Can you work these out from the model? Positions are in its coordinate system, mm. Face numbers are marked on the shaded views. A direction names the side the tool comes from. Give positions to 0.01 mm unless a question says otherwise; leave off trailing zeros. Order: outer loops, then holes, each group sorted by start corner. A loop starts at its lowest first (then second) coordinate and runs counter-clockwise, first axis right, second up. Notation, with made-up numbers: (25.25, 87) - (70.25, 87) arc R5 ccw to (70.25, 94) - close; hole circle Ø2 at (10, 21.25). An arc over 180 degrees is marked (long way). Answer as a JSON object with one key per item and string values.
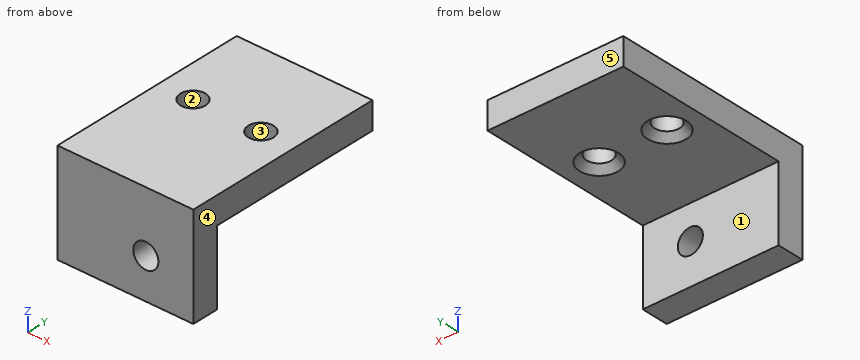
```python
from build123d import *

# Parameters (mm, degrees)
BOSS_EXTRUDE1_DEPTH = 10
SKETCH2_R           = 1.85
CUT_EXTRUDE1_DEPTH  = 30.949958264
BOSS_EXTRUDE2_DEPTH = 10
SKETCH4_R           = 1.85
CUT_EXTRUDE2_DEPTH  = 30.949958264
CHAMFER1_SIZE       = 1


with BuildPart() as part:
    # Sketch1 → Boss-Extrude1 (new body)
    with BuildSketch(Plane(origin=(0, 0, 0), x_dir=(0, 0, -1), z_dir=(1, 0, 0))):
        Polygon((-4, 26), (0, 26), (0, 0), (11, 0), (11, -4), (-4, -4), align=None)
    extrude(amount=BOSS_EXTRUDE1_DEPTH)

    # Sketch2 → Cut-Extrude1 (cut, through all)
    with BuildSketch(Plane(origin=(0, 0, 0), x_dir=(1, 0, 0), z_dir=(0, 1, 0))):
        with Locations(Location((3, 5, 0), (0, 0, 270))):
            Circle(SKETCH2_R)
    extrude(amount=-CUT_EXTRUDE1_DEPTH, mode=Mode.SUBTRACT)

    # Sketch5 → Boss-Extrude2 (add)
    with BuildSketch(Plane.ZY):
        Polygon((-11, -4), (4, -4), (4, 26), (0, 26), (0, 0), (-11, 0), align=None)
    extrude(amount=BOSS_EXTRUDE2_DEPTH)

    # Sketch4 → Cut-Extrude2 (cut, through all)
    with BuildSketch(Plane(origin=(0, 0, 0), x_dir=(-1, 0, 0), z_dir=(0, 0, -1))):
        with Locations((-5, 13)):
            Circle(SKETCH4_R)
        with Locations((5, 13)):
            Circle(SKETCH4_R)
    extrude(amount=-CUT_EXTRUDE2_DEPTH, mode=Mode.SUBTRACT)

    # Chamfer1
    chamfer1_edges = [part.edges().sort_by_distance(p)[0] for p in [
        (6.85, 13, 0),
        (-3.15, 13, 0),
    ]]
    chamfer(chamfer1_edges, length=CHAMFER1_SIZE)


solid = part.part
```
Q1. I need wall thicknesses on L1, parallel to X at y = -2.35, z = -5; L2, parallel to X at y = 12.75, z = 1; L3, parallel to Y at x = -5, z = 2.6. Which ranges of each line are inside material? Lowest first, please.
Recorded:
{"L1": "x = -10 to 1.15, 4.85 to 10", "L2": "x = -10 to -6.83, -3.17 to 3.17, 6.83 to 10", "L3": "y = -4 to 11.15, 14.85 to 26"}
Q2. We'd pull the mould along Y, two halves only. Please class the marked faces 3, 4 and 5: released by +Y, released by -Y, zero draft, split by the parting line, or undercut.
Recorded:
{"face 3": "undercut", "face 4": "zero draft", "face 5": "released by +Y"}
Q3. If we section it at A-A, the plane x = -5: Please give me the cut outline in (y, z), then the cut area to 3 significant figures.
Recorded:
{"outline": "(-4, -11) - (0, -11) - (0, 0) - (10.15, 0) - (11.15, 1) - (11.15, 4) - (-4, 4) - close; (14.85, 1) - (15.85, 0) - (26, 0) - (26, 4) - (14.85, 4) - close", "area": "148 mm^2"}
Q4. If we section it at D-D, the plane z = 3: Please give me the cut outline in (x, y), then the cut area to 3 significant figures.
Recorded:
{"outline": "(-10, -4) - (10, -4) - (10, 26) - (-10, 26) - close; hole circle Ø3.7 at (-5, 13); hole circle Ø3.7 at (5, 13)", "area": "578 mm^2"}
Q5. Which directions (+Z, -Z, +X, -X, +Y, -Y) give clear straight access to the entire face, cutting with the end or side of a thin tool? Please do the marked faces 1 and 2.
Recorded:
{"face 1": "-Z, +X, -X, +Y", "face 2": "+Z, -Z"}
Q6. I'm going to push flat-ended pins straight in: pin 1 Ø10 at (x, y) = (-2.5, 16.5) entering from -Z; pin 2 Ø4 at (x, z) = (-1.5, -3.5) entering from +Y. Where does each tip first touch, or does it pass through?
Recorded:
{"pin 1": "stops at z = 0", "pin 2": "stops at y = 0"}
Q7. If we section it at B-B, the plane y = 13: Please give me the cut outline in (x, z).
Recorded:
{"outline": "(-10, 0) - (-7.85, 0) - (-6.85, 1) - (-6.85, 4) - (-10, 4) - close; (-3.15, 1) - (-2.15, 0) - (2.15, 0) - (3.15, 1) - (3.15, 4) - (-3.15, 4) - close; (6.85, 1) - (7.85, 0) - (10, 0) - (10, 4) - (6.85, 4) - close"}
Q8. If we section it at C-C, the plane z = -5: Please give me the cut outline in (x, y).
Recorded:
{"outline": "(-10, -4) - (1.15, -4) - (1.15, 0) - (-10, 0) - close; (4.85, -4) - (10, -4) - (10, 0) - (4.85, 0) - close"}
